Autodesk Inventor part; units mm, degrees
ref_plane "YZ Plane" through (0, 0, 0) normal (1, 0, 0) x (0, 1, 0)
ref_plane "XZ Plane" through (0, 0, 0) normal (0, 1, 0) x (-1, 0, 0)
ref_plane "XY Plane" through (0, 0, 0) normal (0, 0, 1) x (1, 0, 0)
ref_plane "Work Plane1" through (0, 0, 0) normal (0, 0, 1) x (1, 0, 0)
sketch "Sketch1" plane through (0, 0, 0) normal (0, 0, 1) x (1, 0, 0)
  line L0 (-264.3187, -990.6) -> (264.3188, -990.6)
  line L1 (264.3188, -990.6) -> (264.3188, -952.5)
  line L2 (264.3188, -952.5) -> (-264.3187, -952.5)
  line L3 (-264.3187, -952.5) -> (-264.3187, -990.6)
  point P0 (0, 0)
  dimension "d0" = 528.6375
  dimension "d1" = 38.1
extrude "Extrusion1" add sketch "Sketch1" along normal blind 25.4
sketch "Sketch2" plane through (0, 0, 25.4) normal (0, 0, 1) x (1, 0, 0)
  line L0 (264.3188, -990.6) -> (264.3188, -952.5)
  line L1 (-264.3187, -952.5) -> (264.3188, -952.5)
  line L2 (264.3188, -952.5) -> (264.3188, -965.2)
  line L3 (264.3188, -965.2) -> (-264.3187, -965.2)
  line L4 (-264.3187, -965.2) -> (-264.3187, -952.5)
  point P0 (0, 0)
  dimension "d4" = 12.7
extrude "Extrusion2" cut sketch "Sketch2" against normal blind 8.4646
properties part number "TopBottomBorder"
Model file for the job. Use its own axes, mm. A direction names the side the tool comes from. Round coordinates to 2 decimals unless told otherwise and drop trailing zeros. Write each loop counter-clockwise with the first axis right and the second up, starting at its lowest first coordinate (ties: lowest second). Pieces come first, ordered by that corner, then holes. Notation, with made-up numbers: (63, -13.75) - (92, -13.75) arc R28 cw to (92, 23.25) - close; hole circle Ø8 at (-2, -28). An arc over 180 degrees is marked (long way). Use CSV: the item, a comma, the result in double quotes. Start each with the question number.
Item 1: Drill centre lines: L1, parallel to Y at x = -130, z = 24; L2, parallel to Z at x = 139.5, y = -959. Where is each one in solid material? Low to high. Write a range as [from, to].
Item 2: Band-saw the part on A-A (x = 181.5). Write the cut outline in (y, z).
Item 3: Tool access for faces 1 (the face through (4, -965.2, 21)), 2 (the face through (-4, -971, 0)): list every direction of +Z, -Z, +X, -X, +Y, -Y with a clear straight run to the whole face (end or side of a thin tool).
Item 4: Band-saw the part on B-B (y = -959.5). Write the cut outline in (x, z), and give its area (3 significant figures).
Item 5: Pin check, flat tips, straight feed: P1, Ø7, axis at x = 21.5, z = 21, coming from the +Y side; P2, Ø10, axis at x = -58.5, y = -957.5, coming from the +Z side. Stop position of each tip, or through.
Checked values:
1,L1,"y = [-990.6, -965.2]"
1,L2,"z = [0, 16.94]"
2,outline,"(-990.6, 0) - (-952.5, 0) - (-952.5, 16.94) - (-965.2, 16.94) - (-965.2, 25.4) - (-990.6, 25.4) - close"
3,face 1,"+Z, +X, -X, +Y"
3,face 2,"-Z, +X, -X, +Y, -Y"
4,outline,"(-264.32, 0) - (264.32, 0) - (264.32, 16.94) - (-264.32, 16.94) - close"
4,area,"8,950 mm²"
5,P1,"stops at y = -965.2"
5,P2,"stops at z = 16.94"
